The model under review builds one solid part; all positions refer to its coordinate system, in mm. Face numbers are marked on the shaded views. A direction names the side the tool comes from. Give positions to 0.01 mm unless a question says otherwise; leave off trailing zeros. Write each loop counter-clockwise with the first axis right and the second up, starting at its lowest first coordinate (ties: lowest second). Pieces come first, ordered by that corner, then holes. Notation, with made-up numbers: (8, -10.5) -> (55, -10.5) arc R21 cw to (55, 18.5) -> close; hole circle Ø9 at (-29.75, 25.25). An arc over 180 degrees is marked (long way). Use CSV: the item, a comma, the result in double quotes.
```python
from build123d import *

# Parameters (mm, degrees)
F0_W      = 39
F0_H      = 14
F1_DEPTH  = 3.5
F2_W      = 35
F2_H      = 9.7
F2_W_2    = 30
F2_H_2    = 4.7
F3_DEPTH  = 9
F5_DEPTH  = 22.5
F6_W      = 38.4088279873
F6_H      = 13.5485363163
F7_DEPTH  = 3.5
F8_SIZE   = 2
F9_R      = 3
F10_DEPTH = 39.001


with BuildPart() as f1:
    # F0 (on Top) → F1 (new body)
    with BuildSketch(Plane.XY):
        Rectangle(F0_W, F0_H)
    extrude(amount=F1_DEPTH)

    # F2 (on face) → F3 (join)
    with BuildSketch(Plane.XY.offset(3.5)):
        Rectangle(F2_W, F2_H)
        Rectangle(F2_W_2, F2_H_2, mode=Mode.SUBTRACT)
    extrude(amount=F3_DEPTH)

    # F4 (on Right) → F5 (cut, symmetric)
    with BuildSketch(Plane.YZ):
        Polygon((-4.85, 10.7), (4.85, 12.501087971), (-5.2555450427, 12.884117032), align=None)
    extrude(amount=F5_DEPTH, both=True, mode=Mode.SUBTRACT)

    # F6 (on face) → F7 (join)
    with BuildSketch(Plane(origin=(0, -2.0821921756, 11.2139242658), x_dir=(1, 0, 0), z_dir=(0, -0.1825588214, 0.9831949332))):
        with Locations((-0.0044139937, 2.0591521208)):
            Rectangle(F6_W, F6_H)
    extrude(amount=F7_DEPTH)

    # F8
    f8_edges = [f1.edges().sort_by_distance(p)[0] for p in [
        (-0.004414, -7.357026, 13.794321),
        (19.2, -0.6966, 15.031023),
        (-0.004414, 5.963826, 16.267725),
        (-19.208828, -0.6966, 15.031023),
    ]]
    chamfer(f8_edges, length=F8_SIZE)

    # F9
    f9_edges = [f1.edges().sort_by_distance(p)[0] for p in [
        (19.2, -6.854989, 11.090534),
        (19.2, 6.465863, 13.563939),
        (-19.208828, 6.465863, 13.563939),
        (-19.208828, -6.854989, 11.090534),
    ]]
    fillet(f9_edges, radius=F9_R)

    # F10 (cut, through all): a face of the model
    f10_faces = [f1.faces().sort_by_distance(p)[0] for p in [
        (-19.5, 0, 1.75),
    ]]
    extrude(f10_faces, amount=-F10_DEPTH, mode=Mode.SUBTRACT)


solid = f1.part
```
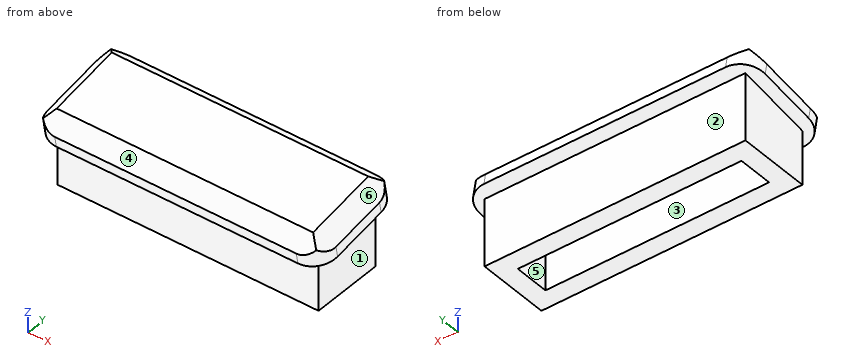
Q1. To check wall thickness, follow probe 1 along Y at (x, z) = (7, 9.25); probe 2 along X at (y, z) = (-0.75, 9.5); probe 3 along Y at (x, z) = (-3.5, 11). State the ranges of each line that lie inside material, in increasing order.
Derived:
probe 1,"y = -4.85 to -2.35, 2.35 to 4.85"
probe 2,"x = -17.5 to -15, 15 to 17.5"
probe 3,"y = -6.84 to -2.35, 2.35 to 4.85"
Q2. Machinability: for the marked faces 1, 2 and 3, which of the approach directions +Z, -Z, +X, -X, +Y, -Y give a long, thin tool a straight path to every point of the face, cutting with its end or side? Answer none if there is none.
Derived:
face 1,"-Z, +X, +Y"
face 2,"-Z, +X, -X, +Y"
face 3,"-Z"
Q3. Consider section D-D (y = -1.25). Write out the cut boundary in (x, z), then the cut area to 3 significant figures.
Derived:
outline,"(-19.21, 11.37) -> (-17.5, 11.37) -> (-17.5, 3.5) -> (-15, 3.5) -> (-15, 11.37) -> (15, 11.37) -> (15, 3.5) -> (17.5, 3.5) -> (17.5, 11.37) -> (19.2, 11.37) -> (19.2, 12.89) -> (17.2, 14.93) -> (-17.21, 14.93) -> (-19.21, 12.89) -> close"
area,"172 mm2"
Q4. Consider section C-C (y = 2). Write out the cut boundary in (x, z), then the cut area to 3 significant figures.
Derived:
outline,"(-19.21, 11.97) -> (-17.5, 11.97) -> (-17.5, 3.5) -> (-15, 3.5) -> (-15, 11.97) -> (15, 11.97) -> (15, 3.5) -> (17.5, 3.5) -> (17.5, 11.97) -> (19.2, 11.97) -> (19.2, 13.5) -> (17.2, 15.53) -> (-17.21, 15.53) -> (-19.21, 13.5) -> close"
area,"175 mm2"
Q5. Insertion check: pin 1 (3 mm diameter, centred on x = -12.5, y = 0.5, fed in from -Z); pin 2 (4 mm diameter, centred on y = 0.5, z = 7, fed in from -X); pin 3 (1.5 mm diameter, centred on y = -4.5, z = 9, fed in from +X). Each pin has a flat end and moves straight along its axis. Give the tip position at first contact, or say it passes through.
Derived:
pin 1,"stops at z = 11.41"
pin 2,"stops at x = -17.5"
pin 3,"stops at x = 17.5"
Q6. Consider section B-B (z = 6.75). Write out the cut boundary in (x, y).
Derived:
outline,"(-17.5, -4.85) -> (17.5, -4.85) -> (17.5, 4.85) -> (-17.5, 4.85) -> close; hole (-15, -2.35) -> (15, -2.35) -> (15, 2.35) -> (-15, 2.35) -> close"
Q7. The part is to be moulded in two halves that separate along X. For the marked faces 4, 5 and 6, say which applies: pulls with the +X half, pulls with the -X half, needs draft (parallel to the pull), parting line crosses it, or undercut.
Derived:
face 4,"needs draft"
face 5,"undercut"
face 6,"pulls with the +X half"
